Geometry: see drawing. Coordinates: mm, zero at the bounding-box minimum. A direction names the side the tool comes from. Give positions to 0.01 mm unless a question says otherwise; leave off trailing zeros. Loops run counter-clockwise (first coordinate to the right, second up) from the corner with the lowest first, then second, coordinate; pieces in that order, holes last. Notation, with made-up numbers: M -20.75,28 L -11.75,28 A8 ccw -11.75,40 Z; hole C 78.5,-14 d8. An arc over 180 degrees is marked long. Use a Markdown table: item, result. Add a question column.
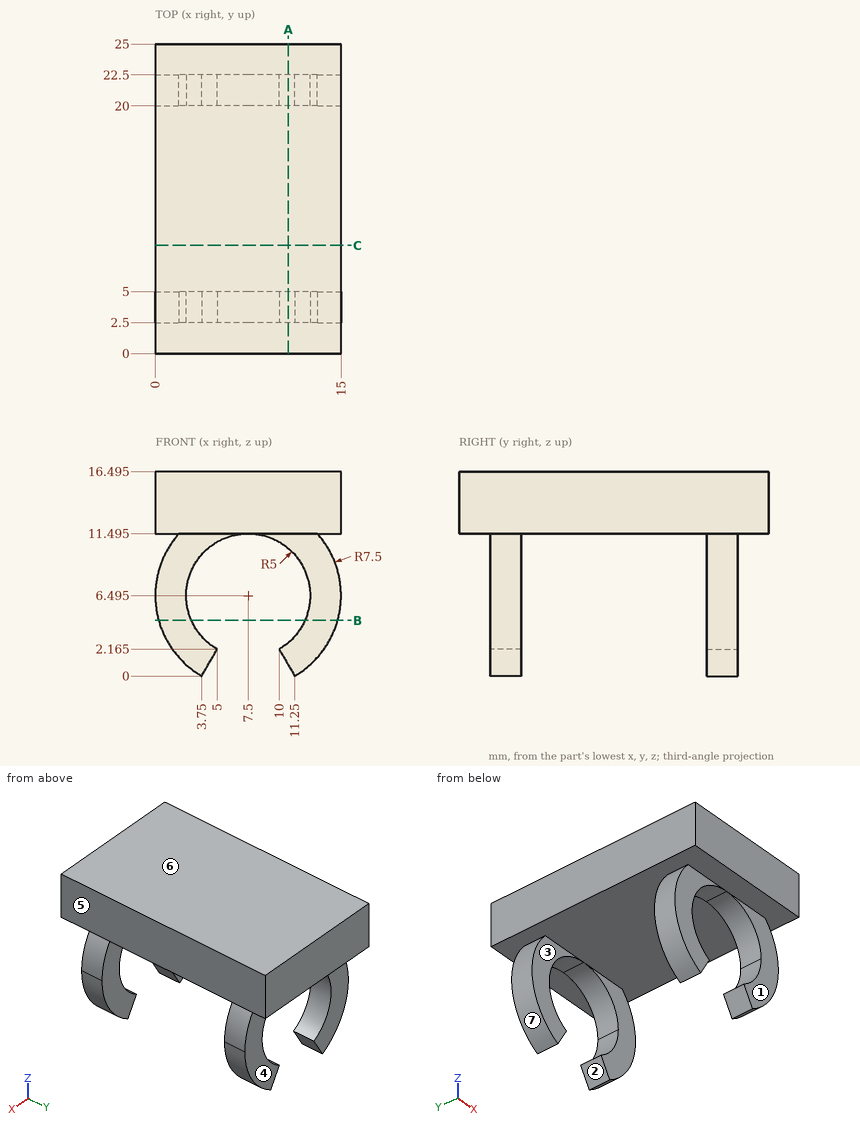
1) Reachability of the marked faces 1, 2, 3 and 4 from +Z, -Z, +X, -X, +Y, -Y: full face, straight path, thin tool, end or side. Return the list, or none.
2) Contact query for flat-ended pins moving along their axis: P1, Ø4, axis at x = 12, z = 5, coming from the -Y side; P2, Ø8.5, axis at x = 11, z = 7, coming from the +Y side; P3, Ø1, axis at x = 9.5, z = 3, coming from the +Y side; P4, Ø4.5, axis at x = 8, y = 17, coming from the -Z side (3 decimals). Output: stop coordinate, or through.
3) Pull-direction query (Z, two-part tool) for the marked faces 5, 6 and 7; classes: pulls with the +Z half, pulls with the -Z half, needs draft (parallel to the pull), parting line crosses it, or undercut.
4) Section query A-A, the plane x = 10.75. Return the cut outline in (y, z) (1 decimal), and give its area (3 significant figures).
5) Section query C-C, the plane y = 8.75. Return the cut outline in (x, z) (1 decimal).
6) Section query B-B, the plane z = 4.5. Return the cut outline in (x, y) (1 decimal).
7) Ray query, line 1 (X direction, y = 21.25, z = 6.25); line 2 (Y direction, x = 13, z = 7.25); line 3 (Z direction, x = 8.75, y = 19.5) (1 decimal). Return the intervals inside material, ascending. Write a range as [from, to].
Entries:
| question | item | result |
|---|---|---|
| 1 | face 1 | -Z, +X, -X, -Y |
| 1 | face 2 | -Z, +Y, -Y |
| 1 | face 3 | -Z, +X, -X |
| 1 | face 4 | -Z, +X, -X, +Y |
| 2 | P1 | stops at y = 2.5 |
| 2 | P2 | stops at y = 22.5 |
| 2 | P3 | passes through |
| 2 | P4 | stops at z = 11.495 |
| 3 | face 5 | needs draft |
| 3 | face 6 | pulls with the +Z half |
| 3 | face 7 | undercut |
| 4 | outline | M 0,11.5 L 2.5,11.5 L 2.5,10.3 L 5,10.3 L 5,11.5 L 20,11.5 L 20,10.3 L 22.5,10.3 L 22.5,11.5 L 25,11.5 L 25,16.5 L 0,16.5 Z; M 2.5,0.9 L 5,0.9 L 5,2.7 L 2.5,2.7 Z; M 20,0.9 L 22.5,0.9 L 22.5,2.7 L 20,2.7 Z |
| 4 | area | 140 mm² |
| 5 | outline | M 0,11.5 L 15,11.5 L 15,16.5 L 0,16.5 Z |
| 6 | outline | M 0.3,2.5 L 2.9,2.5 L 2.9,5 L 0.3,5 Z; M 0.3,20 L 2.9,20 L 2.9,22.5 L 0.3,22.5 Z; M 12.1,2.5 L 14.7,2.5 L 14.7,5 L 12.1,5 Z; M 12.1,20 L 14.7,20 L 14.7,22.5 L 12.1,22.5 Z |
| 7 | line 1 | x = [0, 2.51], [12.49, 15] |
| 7 | line 2 | y = [2.5, 5], [20, 22.5] |
| 7 | line 3 | z = [11.5, 16.5] |
